Design review of the part shown in the three views and the two pictorial views. Dimensions are in mm from the part's minimum x, y and z. Coordinates: 2 decimals unless noted, no trailing zeros. Loops run counter-clockwise (first coordinate to the right, second up) from the corner with the lowest first, then second, coordinate; pieces in that order, holes last. Notation, with made-up numbers: (77.5, 1) - (97.5, 1) arc R15 ccw to (97.5, 12) - close; hole circle Ø11 at (16, -36). An arc over 180 degrees is marked (long way). One line per item, written item: value. Start each with the question number.
1. Take a section at C-C, the plane x = 53. State the section outline as (y, z) points.
2. To check wall thickness, follow line 1 (X direction, y = 14.25, z = 5.5); line 2 (Y direction, x = 159, z = 15.5); line 3 (Y direction, x = 218, z = 17.5). State the ranges of each line that lie inside material, in increasing order. Write a range as from..to.
3. Insertion check: pin 1 (3 mm diameter, centred on y = 24, z = 8.5, fed in from -X); pin 2 (12 mm diameter, centred on y = 20, z = 20.5, fed in from +X); pin 3 (6 mm diameter, centred on y = 23, z = 8.5, fed in from +X); pin 4 (4 mm diameter, centred on x = 247.5, y = 12, fed in from -Z). Each pin has a flat end and moves straight along its axis. Give the tip position at first contact, or say it passes through.
4. Take a section at A-A, the plane y = 15. State the section outline as (x, z) points, and give its area (3 significant figures).
5. Take a section at D-D, the plane y = 27. State the section outline as (x, z) points, and give its area (3 significant figures).
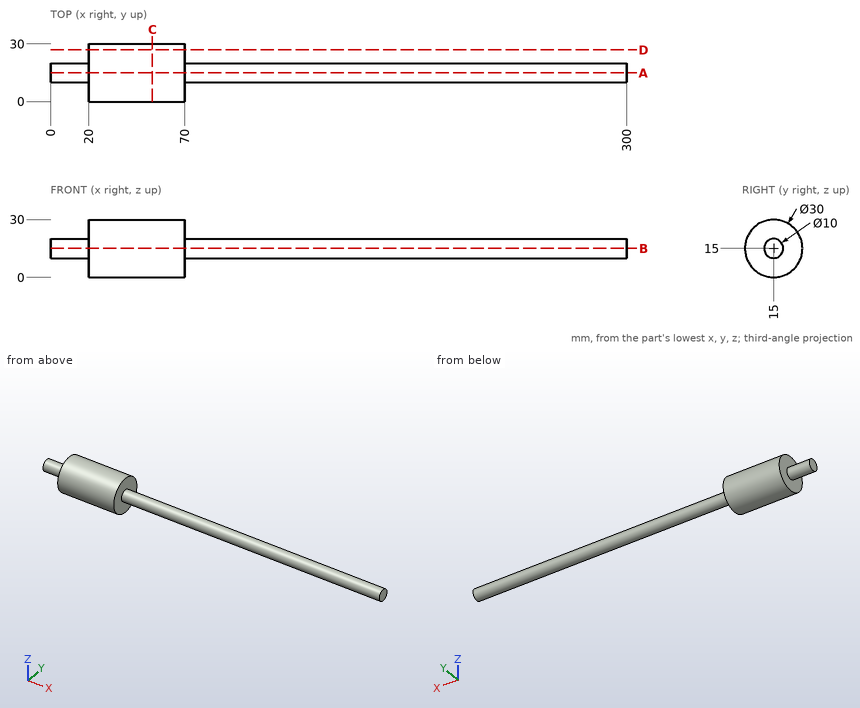
Solutions:
1. outline: circle Ø30 at (15, 15)
2. line 1: 20..70
2. line 2: 10.03..19.97
2. line 3: 10.67..19.33
3. pin 1: x = 20
3. pin 2: x = 300
3. pin 3: x = 70
3. pin 4: z = 10.1
4. outline: (0, 10) - (20, 10) - (20, 0) - (70, 0) - (70, 10) - (300, 10) - (300, 20) - (70, 20) - (70, 30) - (20, 30) - (20, 20) - (0, 20) - close
4. area: 4,000 mm2
5. outline: (20, 6) - (70, 6) - (70, 24) - (20, 24) - close
5. area: 900 mm2
